Autodesk Inventor part; units mm, degrees
ref_plane "YZ Plane" through (0, 0, 0) normal (1, 0, 0) x (0, 1, 0)
ref_plane "XZ Plane" through (0, 0, 0) normal (0, 1, 0) x (-1, 0, 0)
ref_plane "XY Plane" through (0, 0, 0) normal (0, 0, 1) x (1, 0, 0)
sketch "Sketch1" plane through (0, 0, 0) normal (0, 1, 0) x (-1, 0, 0)
  line L0 (-21, 22) -> (21, 22)
  line L1 (21, 22) -> (21, -22)
  line L2 (21, -22) -> (-21, -22)
  line L3 (-21, -22) -> (-21, 22)
  line L4 (-21, 22) -> (21, -22) construction
  line L5 (21, 22) -> (-21, -22) construction
  point P0 (0, 0)
  dimension "d0" = 42
  dimension "d1" = 44
extrude "wall2" add sketch "Sketch1" along normal blind 6.4
sketch "Sketch7" plane through (0, 6.4, 0) normal (0, 1, 0) x (1, 0, 0)
  line L0 (1, -22) -> (1, 22) construction
  line L1 (21, 22) -> (-21, 22)
  line L2 (-21, -22) -> (21, -22)
  line L3 (-21, 12) -> (21, 12) construction
  line L4 (21, -22) -> (21, 22)
  line L5 (-21, 22) -> (-21, -22)
  circle A0 centre (1, 12) radius 5.81
  point P0 (0, 0)
  dimension "d74" = 34
  dimension "d75" = 22
  dimension "d76" = 11.6
extrude "bigcircle" cut sketch "Sketch7" against normal blind 6.4 contours A0
sketch "Sketch8" plane through (0, 6.4, 0) normal (0, 1, 0) x (1, 0, 0)
  line L0 (-21, -22) -> (-21, 22)
  line L1 (-21, 12) -> (21, 12) construction
  line L2 (21, 22) -> (21, -22)
  line L3 (1, 22) -> (1, -22) construction
  line L4 (21, -22) -> (21, 22)
  line L5 (21, 22) -> (-21, 22)
  line L6 (-21, -22) -> (21, -22)
  circle A0 centre (-5, 12) radius 2.96
  point P0 (0, 0)
  dimension "d81" = 22
  dimension "d82" = 34
  dimension "d83" = 5.9
  dimension "d84" = 6
extrude "smallcircle" cut sketch "Sketch8" against normal blind 6.4 contours A0
fillet "Fillet4" radius 2 2 edges at (-4.0829, 3.2, -9.1857) (-4.0829, 3.2, -14.8143)
fillet_without_effect "Fillet5"
fillet "Fillet6" radius 2 1 edges at (-21, 3.2, -22)
fillet "Fillet7" radius 2 1 edges at (21, 3.2, -22)
fillet "Fillet8" radius 2 1 edges at (-21, 3.2, 22)
fillet "Fillet9" radius 2 1 edges at (21, 3.2, 22)
sketch "Sketch9" plane through (0, 6.4, 0) normal (0, 1, 0) x (1, 0, 0)
  line L0 (7.31, 17.1525) -> (7.31, -6.1616) construction
  line L1 (6.81, 14.2171) -> (6.81, 9.0836) construction
  arc A0 (-3.488, 8.3102) -> (-3.488, 15.6898) centre (1, 12) ccw
  line L2 (-21, 12) -> (14.6779, 12) construction
  line L3 (7.31, 10) -> (11.31, 10)
  line L4 (11.31, 10) -> (11.31, 14)
  line L5 (11.31, 14) -> (7.31, 14)
  line L6 (7.31, 14) -> (7.31, 10)
  line L7 (7.31, 10) -> (11.31, 14) construction
  line L8 (11.31, 10) -> (7.31, 14) construction
  line L9 (-21, 20) -> (-21, -20)
  line L10 (-20.49, 14) -> (-16.49, 14)
  line L11 (-16.49, 14) -> (-16.49, 10)
  line L12 (-16.49, 10) -> (-20.49, 10)
  line L13 (-20.49, 10) -> (-20.49, 14)
  line L14 (-20.49, 14) -> (-16.49, 10) construction
  line L15 (-16.49, 14) -> (-20.49, 10) construction
  point P0 (0, 0)
  point P1 (9.31, 12)
  point P2 (-18.49, 12)
  dimension "d93" = 0.5
  dimension "d94" = 4
  dimension "d95" = 23.3
extrude "Extrusion7" add sketch "Sketch9" along normal blind 4
equation "\"d0\" = wallw"
equation "\"d1\" = wallh"
equation "\"d72\" = wall2_thick"
equation "\"d74\" = distancefrombottom"
equation "\"d75\" = distancefromleft"
equation "\"d76\" = servobigcircledia"
equation "\"d79\" = wall2_thick"
equation "\"d81\" = distancefromleft"
equation "\"d82\" = distancefrombottom"
equation "\"d83\" = servosmallcircledia"
equation "\"d85\" = wall2_thick"
equation "\"d89\" = cornerrad"
equation "\"d90\" = cornerrad"
equation "\"d91\" = cornerrad"
equation "\"d92\" = cornerrad"
equation "\"d94\" = servomountsquare"
equation "\"d96\" = servomounth"
equation "\"printer3dtolerance\" = 0.1"
equation "\"wallw\" = 42"
equation "\"wallh\" = 44"
equation "\"cornerrad\" = 2"
equation "\"baseextra\" = 2"
equation "\"wall1_thick\" = 8"
equation "\"wall2_thick\" = 6.4"
equation "\"wall3_thick\" = 4"
equation "\"wall1slot\" = 8.1"
equation "\"wall2slot\" = 6.5"
equation "\"wall3slot\" = 4.1"
equation "\"gap2\" = 28"
equation "\"baseh\" = 79"
equation "\"basew\" = 44"
equation "\"base_thick\" = 6"
equation "\"base_slots_depth\" = 4"
equation "\"servomounth\" = 4"
equation "\"servosmallcircledia\" = 5.9"
equation "\"servomountsquare\" = 4"
equation "\"servobigcircledia\" = 11.6"
equation "\"servo9gw\" = 22.8"
equation "\"distancefromleft\" = 22"
equation "\"servopolygonl\" = 5.9"
equation "\"servopolygonr\" = 6.1"
equation "\"distancefrombottom\" = 34"
equation "\"d49\" = distancefrombottom"
equation "\"adapterh\" = 16"
equation "\"wall3slotd\" = 2"
equation "\"adapterw\" = 32"
equation "\"wall3slotd_1\" = 2"
equation "\"wall3slotw\" = 36"
equation "\"armslotd\" = 2"
equation "\"armthick\" = 3"
equation "\"armw\" = 34"
equation "\"fanhb\" = 11"
equation "\"fanhs\" = 9.6"
equation "\"adapterwallthick\" = 6"
equation "\"adapterwallslotd\" = 2"
equation "\"armhornthick\" = 3"
equation "\"hornscrewholed\" = 2"
equation "\"hornscrewheadd\" = 3"
equation "\"hornthick\" = 1.5"
properties part number "wall-middle" material "Wood (Oak)"
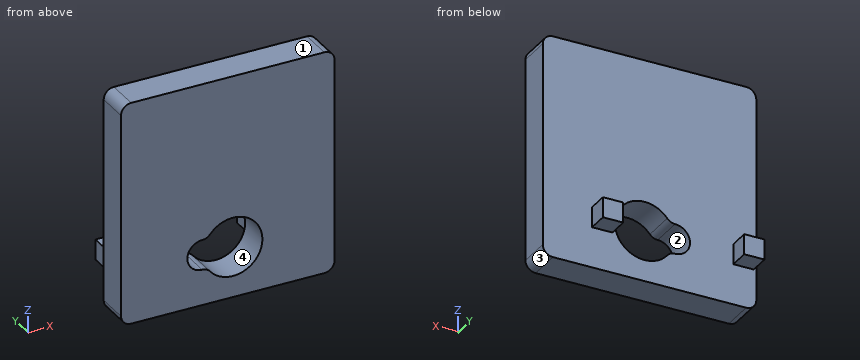
Work out the finished part from the listing and answer in its coordinate system (mm). Face numbers are marked on the shaded views. Round coordinates to 2 decimals unless told otherwise and drop trailing zeros. Loops run counter-clockwise (first coordinate to the right, second up) from the corner with the lowest first, then second, coordinate; pieces in that order, holes last. Notation, with made-up numbers: (54, -24.5) - (103, -24.5) arc R22 ccw to (103, -1.5) - close; hole circle Ø2 at (69.5, 41). An arc over 180 degrees is marked (long way). Use one line per item in the form item = value. Start each with the question number.
(1) Flat-ended cylindrical pins translate along their axes: P1, Ø2, axis at x = -18.5, y = 8.5, coming from the +Z side; P2, Ø3, axis at y = 9, z = -12, coming from the -X side; P3, Ø1.2, axis at y = 9, z = -12.5, coming from the +X side. Find the tip coordinate at first contact, or state that the pin passes through.
(2) Find section A-A on y = 7. Determine the outline of the cut face in (x, z).
(3) Determine the mould class of the marked faces 1, 2, 3 and 4 for opening direction X: +X half, -X half, draft (parallel to the pull), parting line (faces both ways), or undercut.
(4) Consider line 1 (X direction, y = 2.25, z = -12); line 2 (Z direction, x = 1, y = 2.25); line 3 (Y direction, x = -1, z = 12). Determine where each line is inside the solid, lowest interval first.
(5) Find section B-B on x = 1. Determine the outline of the cut face in (y, z).
(6) Find section C-C on z = -4. Determine the outline of the cut face in (x, y).
Answer list:
q1.P1 = -10
q1.P2 = -20.49
q1.P3 = 11.31
q2.outline = (-20.49, -14) - (-16.49, -14) - (-16.49, -10) - (-20.49, -10) - close; (7.31, -14) - (11.31, -14) - (11.31, -10) - (7.31, -10) - close
q3.face_1 = draft
q3.face_2 = undercut
q3.face_3 = +X half
q3.face_4 = undercut
q4.line_1 = -21 to -7.96, 6.81 to 21
q4.line_2 = -22 to -17.81, -6.19 to 22
q4.line_3 = 0 to 6.4
q5.outline = (0, -22) - (6.4, -22) - (6.4, -17.81) - (0, -17.81) - close; (0, -6.19) - (6.4, -6.19) - (6.4, 22) - (0, 22) - close
q6.outline = (-21, 0) - (21, 0) - (21, 6.4) - (-21, 6.4) - close
